from build123d import *

# Parameters (mm, degrees)
SKETCH1_W           = 100
SKETCH1_H           = 50
BOSS_EXTRUDE1_DEPTH = 10
CHAMFER1_SIZE       = 10
CHAMFER2_SIZE       = 10
SKETCH2_W           = 60
SKETCH2_H           = 10
BOSS_EXTRUDE3_DEPTH = 40
CUT_EXTRUDE1_DEPTH  = 64
BOSS_EXTRUDE5_START = 15
BOSS_EXTRUDE5_DEPTH = 15
BOSS_EXTRUDE6_DEPTH = 15


with BuildPart() as part:
    # Sketch1 → Boss-Extrude1 (new body)
    with BuildSketch(Plane(origin=(0, 0, 0), x_dir=(1, 0, 0), z_dir=(0, 1, 0))):
        Rectangle(SKETCH1_W, SKETCH1_H)
    extrude(amount=BOSS_EXTRUDE1_DEPTH)

    # Chamfer1
    chamfer1_edges = [part.edges().sort_by_distance(p)[0] for p in [
        (-50, 10, 0),
    ]]
    chamfer(chamfer1_edges, length=CHAMFER1_SIZE - 0.0001)  # a hair under: the kernel refuses the full size

    # Chamfer2
    chamfer2_edges = [part.edges().sort_by_distance(p)[0] for p in [
        (50, 10, 0),
    ]]
    chamfer(chamfer2_edges, length=CHAMFER2_SIZE - 0.0001)  # a hair under: the kernel refuses the full size

    # Sketch2 → Boss-Extrude3 (add)
    with BuildSketch(Plane(origin=(0, 0, 0), x_dir=(1, 0, 0), z_dir=(0, 1, 0))):
        with Locations((0, -15)):
            Rectangle(SKETCH2_W, SKETCH2_H)
        with Locations((0, 15)):
            Rectangle(SKETCH2_W, SKETCH2_H)
    extrude(amount=BOSS_EXTRUDE3_DEPTH)

    # Sketch4 → Cut-Extrude1 (cut)
    with BuildSketch(Plane.XY.offset(20)):
        with BuildLine():
            Line((-12.5, 40), (12.5, 40))
            ThreePointArc((12.5, 40), (0, 27.5), (-12.5, 40))
        make_face()
    extrude(amount=-CUT_EXTRUDE1_DEPTH, mode=Mode.SUBTRACT)

    # Sketch10 → Boss-Extrude5 (add)
    with BuildSketch(Plane.XY.offset(20).offset(BOSS_EXTRUDE5_START)):
        with BuildLine():
            Line((-25, 40), (-12.5, 40))
            ThreePointArc((-12.5, 40), (0, 27.5), (12.5, 40))
            Line((12.5, 40), (25, 40))
            ThreePointArc((25, 40), (0, 15), (-25, 40))
        make_face()
    extrude(amount=-BOSS_EXTRUDE5_DEPTH)

    # Sketch11 → Boss-Extrude6 (add)
    with BuildSketch(Plane(origin=(0, 0, -20), x_dir=(-1, 0, 0), z_dir=(0, 0, -1))):
        with BuildLine():
            Line((-12.5, 40), (-25, 40))
            ThreePointArc((-25, 40), (0, 15), (25, 40))
            Line((25, 40), (12.5, 40))
            ThreePointArc((12.5, 40), (0, 27.5), (-12.5, 40))
        make_face()
    extrude(amount=BOSS_EXTRUDE6_DEPTH)


solid = part.part
Verification items for the finished model (mm, model axes). A direction names the side the tool comes from. Give positions to 0.01 mm unless a question says otherwise; leave off trailing zeros. Write each loop counter-clockwise with the first axis right and the second up, starting at its lowest first coordinate (ties: lowest second). Pieces come first, ordered by that corner, then holes. Notation, with made-up numbers: M 42.5,-8.5 L 98.5,-8.5 A26 ccw 98.5,21.5 Z; hole C 28,-26.75 d6. An arc over 180 degrees is marked long. Write item = value, one per line.
(1) Go/stop test with flat-tipped pins: pin 1 Ø8 at (y, z) = (27.5, -16) entering from -X; pin 2 Ø10 at (x, z) = (-33.5, -26.5) entering from +Y; pin 3 Ø5 at (y, z) = (27, -16.5) entering from +X. Record where each tip stops, or that it passes through.
Found:
pin_1 = -30
pin_2 = 10
pin_3 = 30
(2) Sectioned sample at C-C (y = 37.5). Record the cut outline in (x, z).
Found:
outline = M -30,-20 L -24.87,-20 L -24.87,-35 L -12.25,-35 L -12.25,-10 L -30,-10 Z; M -30,10 L -12.25,10 L -12.25,35 L -24.87,35 L -24.87,20 L -30,20 Z; M 12.25,-35 L 24.87,-35 L 24.87,-20 L 30,-20 L 30,-10 L 12.25,-10 Z; M 12.25,10 L 30,10 L 30,20 L 24.87,20 L 24.87,35 L 12.25,35 Z
(3) Sectioned sample at A-A (y = 20). Record the cut outline in (x, z).
Found:
outline = M -30,-20 L -15,-20 L -15,-35 L 15,-35 L 15,-20 L 30,-20 L 30,-10 L -30,-10 Z; M -30,10 L 30,10 L 30,20 L 15,20 L 15,35 L -15,35 L -15,20 L -30,20 Z
(4) Material ranges on line 1 (Z direction, x = -23, y = 18.5); line 2 (Z direction, x = 17.5, y = 32); line 3 (X direction, y = 29.5, z = -25), recorded low to high.
Found:
line_1 = -20 to -10, 10 to 20
line_2 = -35 to -10, 10 to 35
line_3 = -22.69 to -6.78, 6.78 to 22.69
(5) Sectioned sample at B-B (x = 0). Record the cut outline in (y, z).
Found:
outline = M 0,-25 L 10,-25 L 10,-20 L 15,-20 L 15,-35 L 27.5,-35 L 27.5,-10 L 10,-10 L 10,10 L 27.5,10 L 27.5,35 L 15,35 L 15,20 L 10,20 L 10,25 L 0,25 Z
(6) Draft check along Z on faces 1 (the face through (0.55, 15.006, 27.605)), 2 (the face through (-1, 10, 0)), 3 (the face through (-1, 5, -25)). Enter one of: released by +Z, released by -Z, zero draft, split by the parting line, or undercut.
Found:
face_1 = zero draft
face_2 = undercut
face_3 = released by -Z
(7) Access from +Z, -Z, +X, -X, +Y, -Y to the whole of each face (thin tool, end or side, straight path). Record for faces 4 (the face through (30, 25, 15)), 5 (the face through (-0.4, 14.8, 20)), 6 (the face through (-1, 5, 25)).
Found:
face_4 = +Z, -Z, +X, +Y
face_5 = +Z
face_6 = +Z, +X, -X, -Y
(8) Sectioned sample at D-D (y = 11.5). Record the cut outline in (x, z).
Found:
outline = M -30,-20 L 30,-20 L 30,-10 L -30,-10 Z; M -30,10 L 30,10 L 30,20 L -30,20 Z
